Can you work these out from the model? Positions are in its coordinate system, mm. A direction names the side the tool comes from. Round coordinates to 2 decimals unless told otherwise and drop trailing zeros. Order: outer loops, then holes, each group sorted by start corner. A loop starts at its lowest first (then second) coordinate and runs counter-clockwise, first axis right, second up. Notation, with made-up numbers: M -39.5,79.5 L -33.5,79.5 A18 cw -33.5,91.5 Z; hole C -17,15.5 d5. An arc over 180 degrees is marked long. Answer as a JSON object with one key per item and string values. Group by question number.
```python
from build123d import *

# Parameters (mm, degrees)
F0_W      = 50
F0_H      = 40
F1_DEPTH  = 15
F2_R      = 5.75
F3_DEPTH  = 2
F4_R      = 2
F5_DEPTH  = 15.001
F6_W      = 45
F6_H      = 24.904493
F7_DEPTH  = 7.5
F8_R      = 5.1
F9_DEPTH  = 2.5
F10_R     = 1.75
F11_DEPTH = 15.001


with BuildPart() as f1:
    # F0 (on Top) → F1 (new body)
    with BuildSketch(Plane.XY):
        with Locations((25, -20)):
            Rectangle(F0_W, F0_H)
    extrude(amount=F1_DEPTH)

    # F2 (on face) → F3 (cut)
    with BuildSketch(Plane.XY.offset(15)):
        with Locations((10, -30)):
            Circle(F2_R)
    extrude(amount=-F3_DEPTH, mode=Mode.SUBTRACT)

    # F4 (on face) → F5 (cut, through all)
    with BuildSketch(Plane.XY.offset(15)):
        with Locations((29.5, -8.755066)):
            Circle(F4_R)
    extrude(amount=-F5_DEPTH, mode=Mode.SUBTRACT)

    # F6 (on face) → F7 (cut)
    with BuildSketch(Plane.XY.offset(15)):
        with Locations((22.5, -12.452246)):
            Rectangle(F6_W, F6_H)
    extrude(amount=-F7_DEPTH, mode=Mode.SUBTRACT)

    # F8 (on face) → F9 (cut)
    with BuildSketch(Plane.XY.offset(13)):
        with Locations((10, -30)):
            Circle(F8_R)
    extrude(amount=-F9_DEPTH, mode=Mode.SUBTRACT)

    # F10 (on face) → F11 (cut, through all)
    with BuildSketch(Plane.XY.offset(15)):
        with Locations((10, -30)):
            Circle(F10_R)
    extrude(amount=-F11_DEPTH, mode=Mode.SUBTRACT)


solid = f1.part
```
1) For pin 1 (6 mm diameter, centred on x = 14, z = 12, fed in from +Y); pin 2 (3 mm diameter, centred on x = 9.5, y = -13.5, fed in from +Z); pin 3 (5 mm diameter, centred on x = 11.5, y = -29, fed in from +Z); pin 4 (3.5 mm diameter, centred on x = 29.5, y = -8.76, fed in from -Z), each with a flat end and sliding along its axis, tell me the tip position at first contact or that it passes through.
2) I need wall thicknesses on line 1 along Y through (x, z) = (29.5, 5.5); line 2 along Z through (x, y) = (21.5, -21); line 3 along Y through (x, z) = (10, 13.5). Which ranges of each line are inside material? Lowest first, please.
3) Which directions (+Z, -Z, +X, -X, +Y, -Y) give clear straight access to the entire face, cutting with the end or side of a thin tool? Please do faces 1 (the face through (22, -12, 7.5)), 2 (the face through (25, 0, 4)), 3 (the face through (8.7, -35.1, 13)).
4) We'd pull the mould along X, two halves only. Please class faces 4 (the face through (9.786, -35.746, 14.014)), 5 (the face through (25, -40, 7)), 6 (the face through (45, -13, 11)): +X half, -X half, draft (parallel to the pull), parting line (faces both ways), or undercut.
5) If we section it at B-B on x = 29.5: Write out the boundary of the cut face in (y, z), plus the area to 3 significant figures.
6) If we section it at D-D on y = -14.5: Write out the boundary of the cut face in (x, z), plus the area to 4 significant figures.
7) If we section it at A-A on z = 8.75: Write out the boundary of the cut face in (x, y), plus the area to 3 significant figures.
8) If we section it at C-C on x = 36.5: Write out the boundary of the cut face in (y, z).
Findings:
{
 "1": {"pin 1": "stops at y = -24.9", "pin 2": "stops at z = 7.5", "pin 3": "stops at z = 10.5", "pin 4": "passes through"},
 "2": {"line 1": "y = -40 to -10.76, -6.76 to 0", "line 2": "z = 0 to 7.5", "line 3": "y = -40 to -35.75"},
 "3": {"face 1": "+Z, -X, +Y", "face 2": "+Z, -Z, +X, -X, +Y", "face 3": "+Z"},
 "4": {"face 4": "undercut", "face 5": "draft", "face 6": "-X half"},
 "5": {"outline": "M -40,0 L -10.76,0 L -10.76,7.5 L -24.9,7.5 L -24.9,15 L -40,15 Z; M -6.76,0 L 0,0 L 0,7.5 L -6.76,7.5 Z", "area": "383 mm^2"},
 "6": {"outline": "M 0,0 L 50,0 L 50,15 L 45,15 L 45,7.5 L 0,7.5 Z", "area": "412.5 mm^2"},
 "7": {"outline": "M 0,-40 L 50,-40 L 50,0 L 45,0 L 45,-24.9 L 0,-24.9 Z; hole C 10,-30 d3.5", "area": "870 mm^2"},
 "8": {"outline": "M -40,0 L 0,0 L 0,7.5 L -24.9,7.5 L -24.9,15 L -40,15 Z"}
}
